Verification items for the finished model (mm, model axes). Round coordinates to 2 decimals unless told otherwise and drop trailing zeros. Order: outer loops, then holes, each group sorted by start corner. A loop starts at its lowest first (then second) coordinate and runs counter-clockwise, first axis right, second up. Notation, with made-up numbers: (28, 58.25) -> (81, 58.25) arc R24 cw to (81, 83.25) -> close; hole circle Ø11 at (42, 21). An arc over 180 degrees is marked (long way). Put each result on its own line as item: value.
```python
from build123d import *

# Parameters (mm, degrees)
BOSS_EXTRUDE1_DEPTH                            = 1.5748
CSK_FOR_M2_FLAT_HEAD_MACHINE_SCREW1_AT_2_COUNT = 2
CSK_FOR_M2_FLAT_HEAD_MACHINE_SCREW1_AT_2_PITCH = 191.697818903
CSK_FOR_M2_FLAT_HEAD_MACHINE_SCREW1_AT_3_COUNT = 2
CSK_FOR_M2_FLAT_HEAD_MACHINE_SCREW1_AT_3_PITCH = 191.697818903
CSK_FOR_M2_FLAT_HEAD_MACHINE_SCREW1_AT_4_COUNT = 2
CSK_FOR_M2_FLAT_HEAD_MACHINE_SCREW1_AT_4_PITCH = 271.101655369
FILLET1_R                                      = 3
CUT_EXTRUDE1_START                             = -1.5748
CUT_EXTRUDE1_DEPTH                             = 1.5748


with BuildPart() as part:
    # Sketch1 → Boss-Extrude1 (new body)
    with BuildSketch(Plane.XY):
        Polygon((3.302181097, 206.697818903), (3.302181097, 129.997818903), (9.822181097, 129.997818903), (9.822181097, 79.997818903), (3.302181097, 79.997818903), (3.302181097, 3.297818903), (206.702181097, 3.297818903), (206.702181097, 79.997818903), (200.182181097, 79.997818903), (200.182181097, 129.997818903), (206.702181097, 129.997818903), (206.702181097, 206.697818903), align=None)
    extrude(amount=BOSS_EXTRUDE1_DEPTH)

    # Sketch3 → CSK for M2 Flat Head Machine Screw1 (revolve, cut)
    with BuildSketch(Plane(origin=(200.848909451, 9.151090549, 1.5748), x_dir=(0, -1, 0), z_dir=(1, 0, 0))):
        Polygon((0, 0), (0, 1.5748), (1.1, 1.5748), (1.1, 0.9), (2, 0), align=None)
    csk_for_m2_flat_head_machine_screw1 = revolve(axis=Axis((200.848909451, 9.151090549, 7.9248), (0, 0, -1)), mode=Mode.SUBTRACT)

    # CSK for M2 Flat Head Machine Screw1 at 2: CSK for M2 Flat Head Machine Screw1 ×2
    with Locations(*[(-i * CSK_FOR_M2_FLAT_HEAD_MACHINE_SCREW1_AT_2_PITCH, 0, 0) for i in range(1, CSK_FOR_M2_FLAT_HEAD_MACHINE_SCREW1_AT_2_COUNT)]):
        add(csk_for_m2_flat_head_machine_screw1, mode=Mode.SUBTRACT)

    # CSK for M2 Flat Head Machine Screw1 at 3: CSK for M2 Flat Head Machine Screw1 ×2
    with Locations(*[(0, i * CSK_FOR_M2_FLAT_HEAD_MACHINE_SCREW1_AT_3_PITCH, 0) for i in range(1, CSK_FOR_M2_FLAT_HEAD_MACHINE_SCREW1_AT_3_COUNT)]):
        add(csk_for_m2_flat_head_machine_screw1, mode=Mode.SUBTRACT)

    # CSK for M2 Flat Head Machine Screw1 at 4: CSK for M2 Flat Head Machine Screw1 ×2
    with Locations(*[Vector(-0.707106781, 0.707106781, 0) * (i * CSK_FOR_M2_FLAT_HEAD_MACHINE_SCREW1_AT_4_PITCH) for i in range(1, CSK_FOR_M2_FLAT_HEAD_MACHINE_SCREW1_AT_4_COUNT)]):
        add(csk_for_m2_flat_head_machine_screw1, mode=Mode.SUBTRACT)

    # Fillet1
    fillet1_edges = [part.edges().sort_by_distance(p)[0] for p in [
        (206.702181097, 206.697818903, 0.7874),
        (200.182181097, 129.997818903, 0.7874),
        (200.182181097, 79.997818903, 0.7874),
        (206.702181097, 3.297818903, 0.7874),
        (3.302181097, 3.297818903, 0.7874),
        (9.822181097, 79.997818903, 0.7874),
        (9.822181097, 129.997818903, 0.7874),
        (3.302181097, 206.697818903, 0.7874),
    ]]
    fillet(fillet1_edges, radius=FILLET1_R)

    # Sketch4 → Cut-Extrude1 (cut)
    with BuildSketch(Plane.XY.offset(1.5748).offset(CUT_EXTRUDE1_START)):
        with BuildLine():
            Line((6.302181097, 3.297818903), (203.702181097, 3.297818903))
            ThreePointArc((203.702181097, 3.297818903), (205.823501441, 4.176498559), (206.702181097, 6.297818903))
            Line((206.702181097, 6.297818903), (206.702181097, 203.697818903))
            ThreePointArc((206.702181097, 203.697818903), (205.823501441, 205.819139246), (203.702181097, 206.697818903))
            Line((203.702181097, 206.697818903), (6.302181097, 206.697818903))
            ThreePointArc((6.302181097, 206.697818903), (4.180860754, 205.819139246), (3.302181097, 203.697818903))
            Line((3.302181097, 203.697818903), (3.302181097, 6.297818903))
            ThreePointArc((3.302181097, 6.297818903), (4.180860754, 4.176498559), (6.302181097, 3.297818903))
        make_face()
        with BuildLine():
            Line((6.302181097, 3.797818903), (203.702181097, 3.797818903))
            ThreePointArc((203.702181097, 3.797818903), (205.46994805, 4.53005195), (206.202181097, 6.297818903))
            Line((206.202181097, 6.297818903), (206.202181097, 203.697818903))
            ThreePointArc((206.202181097, 203.697818903), (205.46994805, 205.465585856), (203.702181097, 206.197818903))
            Line((203.702181097, 206.197818903), (6.302181097, 206.197818903))
            ThreePointArc((6.302181097, 206.197818903), (4.534414144, 205.465585856), (3.802181097, 203.697818903))
            Line((3.802181097, 203.697818903), (3.802181097, 6.297818903))
            ThreePointArc((3.802181097, 6.297818903), (4.534414144, 4.53005195), (6.302181097, 3.797818903))
        make_face(mode=Mode.SUBTRACT)
    extrude(amount=CUT_EXTRUDE1_DEPTH, mode=Mode.SUBTRACT)


solid = part.part
```
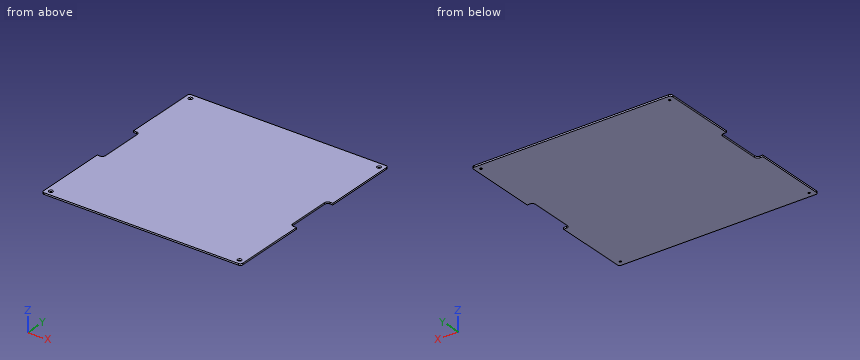
Item 1: Sectioned sample at A-A, the plane z = 0.3. Record the boundary of the cut face in (x, y).
Geometry check:
outline: (3.8, 6.3) arc R2.5 ccw to (6.3, 3.8) -> (203.7, 3.8) arc R2.5 ccw to (206.2, 6.3) -> (206.2, 80) -> (203.18, 80) arc R3 cw to (200.18, 83) -> (200.18, 127) arc R3 cw to (203.18, 130) -> (206.2, 130) -> (206.2, 203.7) arc R2.5 ccw to (203.7, 206.2) -> (6.3, 206.2) arc R2.5 ccw to (3.8, 203.7) -> (3.8, 130) -> (6.82, 130) arc R3 cw to (9.82, 127) -> (9.82, 83) arc R3 cw to (6.82, 80) -> (3.8, 80) -> close; hole circle Ø2.2 at (9.15, 9.15); hole circle Ø2.2 at (9.15, 200.85); hole circle Ø2.2 at (200.85, 9.15); hole circle Ø2.2 at (200.85, 200.85)
Item 2: Depth check by flat-ended pin: pin 1 Ø0.5 at (x, z) = (205, 1) entering from -Y; pin 2 Ø0.8 at (x, z) = (205, 1) entering from +Y; pin 3 Ø0.5 at (y, z) = (95, 0.5) entering from -X. Enter the tip coordinate at first touch or a pass-through.
Geometry check:
pin 1: y = 4.03
pin 2: y = 206.03
pin 3: x = 9.82
Item 3: Material ranges on line 1 along X through (y, z) = (93, 1.5), recorded low to high.
Geometry check:
line 1: 9.82 to 200.18
Item 4: Sectioned sample at B-B, the plane y = 94. Record the boundary of the cut face in (x, z), then the cut area to 3 significant figures.
Geometry check:
outline: (9.82, 0) -> (200.18, 0) -> (200.18, 1.57) -> (9.82, 1.57) -> close
area: 300 mm2
